Read the model definition and answer for the solid it produces. Units are mm, in the model's axes. Give positions to 0.01 mm unless a question says otherwise; leave off trailing zeros. Loops run counter-clockwise (first coordinate to the right, second up) from the corner with the lowest first, then second, coordinate; pieces in that order, holes last. Notation, with made-up numbers: (-5, -12.75) -> (20, -12.75) arc R6 ccw to (20, -2.75) -> close; hole circle Ø8 at (-15.75, 85). An arc over 180 degrees is marked (long way). One line per item, written item: value. Start each with the question number.
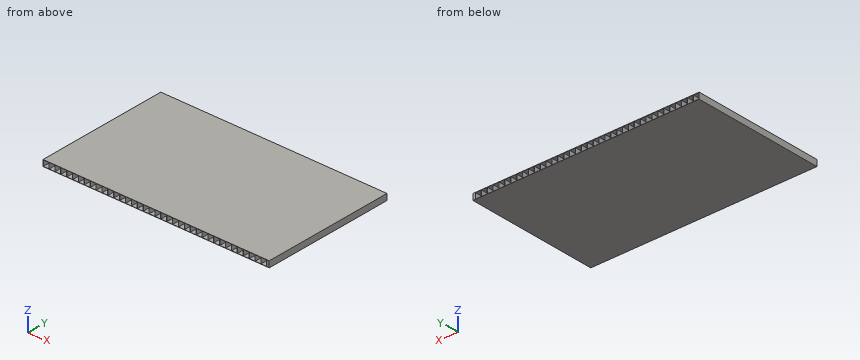
from build123d import *

# Parameters (mm, degrees)
SKETCH1_W           = 221
SKETCH1_H           = 6
SKETCH1_W_2         = 5.5
SKETCH1_H_2         = 5.5
BOSS_EXTRUDE1_DEPTH = 130


with BuildPart() as part:
    # Sketch1 → Boss-Extrude1 (new body)
    with BuildSketch(Plane(origin=(0, 0, 0), x_dir=(1, 0, 0), z_dir=(0, 1, 0))):
        with Locations((110.5, 3)):
            Rectangle(SKETCH1_W, SKETCH1_H)
        with Locations((8.75, 3)):
            Rectangle(SKETCH1_W_2, SKETCH1_H_2, mode=Mode.SUBTRACT)
        with Locations((3, 3)):
            Rectangle(SKETCH1_W_2, SKETCH1_H_2, mode=Mode.SUBTRACT)
        with Locations((14.5, 3)):
            Rectangle(SKETCH1_W_2, SKETCH1_H_2, mode=Mode.SUBTRACT)
        with Locations((20.25, 3)):
            Rectangle(SKETCH1_W_2, SKETCH1_H_2, mode=Mode.SUBTRACT)
        with Locations((26, 3)):
            Rectangle(SKETCH1_W_2, SKETCH1_H_2, mode=Mode.SUBTRACT)
        with Locations((31.75, 3)):
            Rectangle(SKETCH1_W_2, SKETCH1_H_2, mode=Mode.SUBTRACT)
        with Locations((37.5, 3)):
            Rectangle(SKETCH1_W_2, SKETCH1_H_2, mode=Mode.SUBTRACT)
        with Locations((43.25, 3)):
            Rectangle(SKETCH1_W_2, SKETCH1_H_2, mode=Mode.SUBTRACT)
        with Locations((49, 3)):
            Rectangle(SKETCH1_W_2, SKETCH1_H_2, mode=Mode.SUBTRACT)
        with Locations((54.75, 3)):
            Rectangle(SKETCH1_W_2, SKETCH1_H_2, mode=Mode.SUBTRACT)
        with Locations((60.5, 3)):
            Rectangle(SKETCH1_W_2, SKETCH1_H_2, mode=Mode.SUBTRACT)
        with Locations((66.25, 3)):
            Rectangle(SKETCH1_W_2, SKETCH1_H_2, mode=Mode.SUBTRACT)
        with Locations((72, 3)):
            Rectangle(SKETCH1_W_2, SKETCH1_H_2, mode=Mode.SUBTRACT)
        with Locations((77.75, 3)):
            Rectangle(SKETCH1_W_2, SKETCH1_H_2, mode=Mode.SUBTRACT)
        with Locations((83.5, 3)):
            Rectangle(SKETCH1_W_2, SKETCH1_H_2, mode=Mode.SUBTRACT)
        with Locations((89.25, 3)):
            Rectangle(SKETCH1_W_2, SKETCH1_H_2, mode=Mode.SUBTRACT)
        with Locations((95, 3)):
            Rectangle(SKETCH1_W_2, SKETCH1_H_2, mode=Mode.SUBTRACT)
        with Locations((100.75, 3)):
            Rectangle(SKETCH1_W_2, SKETCH1_H_2, mode=Mode.SUBTRACT)
        with Locations((106.5, 3)):
            Rectangle(SKETCH1_W_2, SKETCH1_H_2, mode=Mode.SUBTRACT)
        with Locations((112.25, 3)):
            Rectangle(SKETCH1_W_2, SKETCH1_H_2, mode=Mode.SUBTRACT)
        with Locations((118, 3)):
            Rectangle(SKETCH1_W_2, SKETCH1_H_2, mode=Mode.SUBTRACT)
        with Locations((123.75, 3)):
            Rectangle(SKETCH1_W_2, SKETCH1_H_2, mode=Mode.SUBTRACT)
        with Locations((129.5, 3)):
            Rectangle(SKETCH1_W_2, SKETCH1_H_2, mode=Mode.SUBTRACT)
        with Locations((135.25, 3)):
            Rectangle(SKETCH1_W_2, SKETCH1_H_2, mode=Mode.SUBTRACT)
        with Locations((141, 3)):
            Rectangle(SKETCH1_W_2, SKETCH1_H_2, mode=Mode.SUBTRACT)
        with Locations((146.75, 3)):
            Rectangle(SKETCH1_W_2, SKETCH1_H_2, mode=Mode.SUBTRACT)
        with Locations((152.5, 3)):
            Rectangle(SKETCH1_W_2, SKETCH1_H_2, mode=Mode.SUBTRACT)
        with Locations((158.25, 3)):
            Rectangle(SKETCH1_W_2, SKETCH1_H_2, mode=Mode.SUBTRACT)
        with Locations((164, 3)):
            Rectangle(SKETCH1_W_2, SKETCH1_H_2, mode=Mode.SUBTRACT)
        with Locations((169.75, 3)):
            Rectangle(SKETCH1_W_2, SKETCH1_H_2, mode=Mode.SUBTRACT)
        with Locations((175.5, 3)):
            Rectangle(SKETCH1_W_2, SKETCH1_H_2, mode=Mode.SUBTRACT)
        with Locations((181.25, 3)):
            Rectangle(SKETCH1_W_2, SKETCH1_H_2, mode=Mode.SUBTRACT)
        with Locations((187, 3)):
            Rectangle(SKETCH1_W_2, SKETCH1_H_2, mode=Mode.SUBTRACT)
        with Locations((192.75, 3)):
            Rectangle(SKETCH1_W_2, SKETCH1_H_2, mode=Mode.SUBTRACT)
        with Locations((198.5, 3)):
            Rectangle(SKETCH1_W_2, SKETCH1_H_2, mode=Mode.SUBTRACT)
        with Locations((204.25, 3)):
            Rectangle(SKETCH1_W_2, SKETCH1_H_2, mode=Mode.SUBTRACT)
        with Locations((210, 3)):
            Rectangle(SKETCH1_W_2, SKETCH1_H_2, mode=Mode.SUBTRACT)
        with Locations((215.75, 3)):
            Rectangle(SKETCH1_W_2, SKETCH1_H_2, mode=Mode.SUBTRACT)
    extrude(amount=BOSS_EXTRUDE1_DEPTH)


solid = part.part
Item 1: Consider L1, parallel to Z at x = 60.5, y = 45. Determine where the line is inside the solid, lowest interval first. Write a range as [from, to].
Item 2: A flat-ended cylindrical pin translates along its axis: pin 1 (3 mm diameter, centred on y = 89.5, z = -2, fed in from -X). Find the tip coordinate at first contact, or state that the pin passes through.
Item 3: Section A-A, the plane x = 112 is taken. Determine the outline of the cut face in (y, z).
Item 4: Section B-B, the plane y = 45.5 is taken. State how many separate pieces and enclosed holes the cut face has, plus the area to 4 significant figures.
Computed values:
1. L1: [-6, -5.75], [-0.25, 0]
2. pin 1: x = 0
3. outline: (0, -6) -> (130, -6) -> (130, -5.75) -> (0, -5.75) -> close; (0, -0.25) -> (130, -0.25) -> (130, 0) -> (0, 0) -> close
4. separate pieces: 1
4. enclosed holes: 38
4. area: 176.5 mm²
